Can you work these out from the model? Positions are in its coordinate system, mm. Face numbers are marked on the shaded views. A direction names the side the tool comes from. Give positions to 0.01 mm unless a question says otherwise; leave off trailing zeros. Write each loop counter-clockwise with the first axis right and the second up, starting at its lowest first coordinate (ties: lowest second). Pieces come first, ordered by that corner, then holes.
Autodesk Inventor part; units mm, degrees
ref_plane "Work Plane1" through (0, 6.35, 0) normal (0, 1, 0) x (-1, 0, 0)
ref_plane "YZ Plane" through (0, 0, 0) normal (1, 0, 0) x (0, 1, 0)
ref_plane "XY Plane" through (0, 0, 0) normal (0, 0, 1) x (1, 0, 0)
sketch "Sketch1" plane through (0, 0, 0) normal (0, 0, 1) x (1, 0, 0)
  circle A0 centre (0, 0) radius 6.35
  dimension "d0" = 12.7
extrude "Extrusion1" add sketch "Sketch1" against normal blind 7.1374
sketch "Sketch2" plane through (0, 0, 0) normal (0, 0, 1) x (1, 0, 0)
  circle A0 centre (0, 0) radius 6.35
  circle A1 centre (0, 0) radius 3.175
  dimension "d3" = 6.35
extrude "Extrusion2" cut sketch "Sketch2" against normal up to next contours A1
chamfer "Chamfer1" distance 0.3969 angle 45 4 edges at (-6.35, 0, 0) (-6.35, 0, -7.1374) (-3.175, 0, 0) (-3.175, 0, -7.1374)
ref_plane "Work Plane1" through (0, 6.35, 0) normal (0, 1, 0) x (-1, 0, 0)
sketch "Sketch3" plane through (0, 6.35, 0) normal (0, 1, 0) x (-1, 0, 0)
  line L0 (5.9531, -7.1374) -> (-5.9531, -7.1374)
  line L1 (6.35, -0.3969) -> (6.35, -6.7405)
  point P0 (0, 0)
  point P1 (0, -3.5687)
hole "Hole1" at (0, 6.35, -3.5687) direction (0, -1, 0) diameter 3.302 end up to surface
properties part number "Misc_ShaftCollar_Ruland_SC-4-F" material "Steel, Carbon"
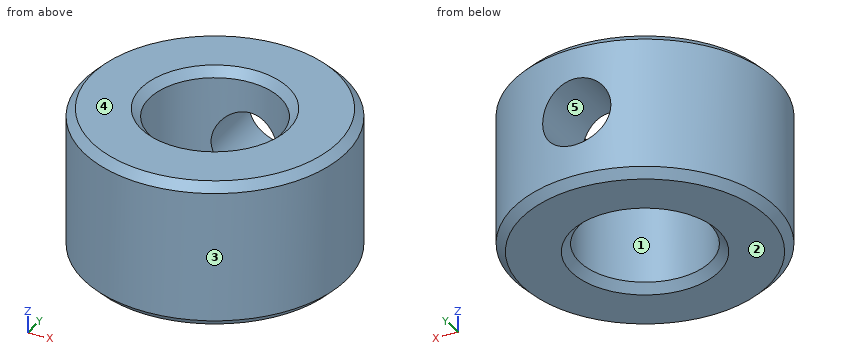
1) For the marked faces 4 and 5, which set-ups out of +Z, -Z, +X, -X, +Y, -Y let a thin tool reach every point of the face, with its end or its side?
Values follow:
face 4: +Z, +X, -X, +Y, -Y
face 5: +Y
2) If we mould it in two halves opening along Y, with no side actions, what happens to the marked faces 1, 2 and 3? For each: +Y half, -Y half, draft (parallel to the pull), parting line (faces both ways), or undercut.
Values follow:
face 1: undercut
face 2: draft
face 3: parting line
3) Suppose I cut it at D-D on z = -2.5. Write out the boundary of the cut face in (x, y) (3 decimals).
Values follow:
outline: (-1.258, 2.915) - (-1.258, 6.224) arc R6.35 ccw (long way) to (1.258, 6.224) - (1.258, 2.915) arc R3.175 cw (long way) to start
4) For pin 1 Ø1 at (y, z) = (2.5, -4) entering from +X, with a flat end and sliding along its axis, tell me the tip position at first contact or that it passes through.
Values follow:
pin 1: stops at x = 6.03
5) Suppose I cut it at A-A on x = 0. State how many separate pieces and enclosed holes the cut face has, plus the area to 3 significant figures.
Values follow:
separate pieces: 3
enclosed holes: 0
area: 34.2 mm2
6) Suppose I cut it at C-C on z = -1.75. Write out the boundary of the cut face in (x, y) (3 decimals), plus the area to 3 significant figures.
Values follow:
outline: circle Ø12.7 at (0, 0); hole circle Ø6.35 at (0, 0)
area: 95.0 mm2
7) Please list where these lines run through material, in increasing order: L1, parallel to Y at x = 0, z = -5.5 (3 decimals); L2, parallel to Z at x = 0, y = 3.8; L3, parallel to Y at x = 0, z = -4.25 (3 decimals).
Values follow:
L1: y = -6.35 to -3.175, 3.175 to 6.35
L2: z = -7.14 to -5.22, -1.92 to 0
L3: y = -6.35 to -3.175
